```python
from build123d import *

# Parameters (mm, degrees)
SKETCH_1_R               = 7.5
SKETCH_1_R_2             = 1.5
EXTRUDE_1_DEPTH          = 20
EXTRUDE_START            = -5.126128
SKETCH_5_R               = 3
EXTRUDE_3_DEPTH          = 13.126128
PATTERN_CIRCULAR_1_COUNT = 6
SKETCH_6_R               = 7.5
CUT_EXTRUDE_1_DEPTH      = 5


with BuildPart() as part:
    # Sketch 1 → Extrude 1 (new body)
    with BuildSketch(Plane.XY):
        Circle(SKETCH_1_R)
        Circle(SKETCH_1_R_2, mode=Mode.SUBTRACT)
    extrude(amount=EXTRUDE_1_DEPTH)



with BuildPart() as body_2:
    # Sketch 2 → Revolve 2 (revolve)
    with BuildSketch(Plane(origin=(0, 0, 0), x_dir=(1, 0, 0), z_dir=(0, 1, 0))):
        Polygon((-30, 0), (-20, 0), (-20, -20), (-30, -20), (-30, -16.5), (-22.5, -16.5), (-22.5, -14.5), (-30, -14.5), (-30, -11), (-22.5, -11), (-22.5, -9), (-30, -9), (-30, -5.5), (-22.5, -5.5), (-22.5, -3.5), (-30, -3.5), align=None)
    revolve(axis=Axis((0, 0, -16.060558383), (0, 0, 1)))


with BuildPart() as part_1:
    add(part.part)

    add(body_2.part)  # Extrude 3 merges body 2
    # Sketch 5 → Extrude 3 (add)
    with BuildSketch(Plane(origin=(0, 12, 0), x_dir=(1, 0, 0), z_dir=(0, 1, 0)).offset(EXTRUDE_START)):
        with Locations((0, -10)):
            Circle(SKETCH_5_R)
    extrude_3 = extrude(amount=EXTRUDE_3_DEPTH)

    # Pattern Circular 1: Extrude 3 ×6 about axis
    pattern_circular_1_axis = Axis((0, 0, 20), (0, 0, -1))
    for i in range(1, PATTERN_CIRCULAR_1_COUNT):
        add(extrude_3.rotate(pattern_circular_1_axis, i * 360 / PATTERN_CIRCULAR_1_COUNT))

    # Sketch 6 → Cut-Extrude 1 (cut)
    with BuildSketch(Plane.XY.offset(20)):
        Circle(SKETCH_6_R)
    extrude(amount=-CUT_EXTRUDE_1_DEPTH, mode=Mode.SUBTRACT)


solid = part_1.part
```
Check sheet for the modelled part. Datum: model origin and axes. Units: mm. A direction names the side the tool comes from. Round coordinates to 2 decimals unless told otherwise and drop trailing zeros. Loops run counter-clockwise (first coordinate to the right, second up) from the corner with the lowest first, then second, coordinate; pieces in that order, holes last. Notation, with made-up numbers: (-33, 86) -> (13, 86) arc R23 cw to (13, 98) -> close; hole circle Ø6 at (62, 51). An arc over 180 degrees is marked (long way). Write item = value, one per line. Start each with the question number.
1) Sectioned sample at C-C, the plane z = 17.75. Record the cut outline in (x, y), plus the area to 3 significant figures.
2) Thickness scan on probe 1 along Y at (x, z) = (0, 4); probe 2 along Z at (x, y) = (-22.5, 9); probe 3 along Y at (x, z) = (0, 9.5). Record the ranges inside material, lowest first.
3) Gauge pin test, flat ends, axial feed: pin 1 Ø3 at (y, z) = (-12.5, 7) entering from +X; pin 2 Ø4.5 at (x, y) = (0, -2) entering from +Z; pin 3 Ø5 at (y, z) = (-22.5, 15.5) entering from -X; pin 4 Ø3 at (x, y) = (5, 9.5) entering from +Z. Record the tip position at first contact, or that the pin passes through.
4) Release check for a two-part mould opening along Z. For faces 4 (the flat face through (4.3, -22.4, 14.5)), 5 (the flat face through (6, 20, 20)), 6 (the cylindrical face through (-1.5, 0.07, 7.4)) record: released by +Z, released by -Z, zero draft, split by the parting line, or undercut.
5) Sectioned sample at B-B, the plane y = 0. State how many separate pieces and enclosed holes the cut face has, plus the area to 3 significant figures.
6) Set-up check for faces 1 (the flat face through (2, 0, 0)), 2 (the flat face through (2, 0, 15)), 3 (the cylindrical face through (0, -13, 7)): record each of +Z, -Z, +X, -X, +Y, -Y from which the full face is reachable in a straight line by a thin tool's end or side.
7) Sectioned sample at A-A, the plane x = -25. Record the cut outline in (y, z).
8) Sectioned sample at D-D, the plane y = -21. Record the cut outline in (x, z), plus the area to 3 significant figures.
Results are:
q1.outline = circle Ø60 at (0, 0); hole circle Ø40 at (0, 0)
q1.area = 1,570 mm^2
q2.probe_1 = -22.5 to -20, -7.5 to -1.5, 1.5 to 7.5, 20 to 22.5
q2.probe_2 = 0 to 3.5, 5.5 to 9, 11 to 14.5, 16.5 to 20
q2.probe_3 = -22.5 to -1.5, 1.5 to 22.5
q3.pin_1 = 27.91
q3.pin_2 = 15
q3.pin_3 = -22.17
q3.pin_4 = through
q4.face_4 = undercut
q4.face_5 = released by +Z
q4.face_6 = zero draft
q5.separate_pieces = 4
q5.enclosed_holes = 0
q5.area = 490 mm^2
q6.face_1 = -Z, +X, -X, +Y, -Y
q6.face_2 = +Z
q6.face_3 = none
q7.outline = (-16.58, 0) -> (16.58, 0) -> (16.58, 3.5) -> (-16.58, 3.5) -> close; (-16.58, 5.5) -> (16.58, 5.5) -> (16.58, 9) -> (-16.58, 9) -> close; (-16.58, 11) -> (16.58, 11) -> (16.58, 14.5) -> (-16.58, 14.5) -> close; (-16.58, 16.5) -> (16.58, 16.5) -> (16.58, 20) -> (-16.58, 20) -> close
q8.outline = (-21.42, 0) -> (21.42, 0) -> (21.42, 3.5) -> (8.08, 3.5) -> (8.08, 5.5) -> (21.42, 5.5) -> (21.42, 9) -> (8.08, 9) -> (8.08, 11) -> (21.42, 11) -> (21.42, 14.5) -> (8.08, 14.5) -> (8.08, 16.5) -> (21.42, 16.5) -> (21.42, 20) -> (-21.42, 20) -> (-21.42, 16.5) -> (-8.08, 16.5) -> (-8.08, 14.5) -> (-21.42, 14.5) -> (-21.42, 11) -> (-8.08, 11) -> (-8.08, 9) -> (-21.42, 9) -> (-21.42, 5.5) -> (-8.08, 5.5) -> (-8.08, 3.5) -> (-21.42, 3.5) -> close
q8.area = 697 mm^2
